Part model, mm, in its own coordinate system. Face numbers are marked on the shaded views. A direction names the side the tool comes from. Coordinates: 2 decimals unless noted, no trailing zeros. Order: outer loops, then holes, each group sorted by start corner. A loop starts at its lowest first (then second) coordinate and runs counter-clockwise, first axis right, second up. Notation, with made-up numbers: (42, 28.5) - (56, 28.5) arc R26 ccw to (56, 50.5) - close; hole circle Ø11 at (70, 3.25). An arc over 180 degrees is marked (long way). Use a Markdown table: item, result. Add a question column.
1) Saw through at D-D on x = 7. List the corners of the cut face in (y, z).
2) Saw through at C-C on y = 3.5. List the corners of the cut face in (x, z), then the cut area to 3 significant figures.
3) Drop flat-ended pins along their axis: P1, Ø2, axis at x = 20, y = 1.5, coming from the +Z side; P2, Ø5, axis at x = 38, y = -2, coming from the -Z side; P3, Ø3, axis at y = -8, z = 0, coming from the +X side; P4, Ø10, axis at x = 22.5, z = -8, coming from the -Y side. Give the stop position or say it passes through.
4) Wall check: L1, parallel to Y at x = 2.55, z = 0; L2, parallel to X at y = -7.5, z = -4; L3, parallel to Z at x = 9.5, y = -1.25. Give the ranges that are in metal, low to high. Write a range as [from, to].
5) Tool access for the marked faces 1, 2 and 3: list every direction of +Z, -Z, +X, -X, +Y, -Y with a clear straight run to the whole face (end or side of a thin tool).
6) Saw through at B-B on y = 0. List the corners of the cut face in (x, z).
7) Saw through at A-A on z = 0. List the corners of the cut face in (x, y), then the cut area to 3 significant figures.
```python
from build123d import *

# Parameters (mm, degrees)
SKETCH1_R           = 1.5
BOSS_EXTRUDE1_DEPTH = 4
SKETCH1_2_R         = 1.5
BOSS_EXTRUDE2_DEPTH = 43
CUT_EXTRUDE1_REACH  = 45
SKETCH2_R           = 1.5


with BuildPart() as part:
    # Sketch1 → Boss-Extrude1 (new body)
    with BuildSketch(Plane(origin=(0, 0, 0), x_dir=(0, 0, -1), z_dir=(1, 0, 0))):
        with BuildLine():
            Line((-4.5, -4.5), (-4.5, 3))
            ThreePointArc((-4.5, 3), (0, 7.5), (4.5, 3))
            Line((4.5, 3), (4.5, -4.5))
            Line((4.5, -4.5), (11.053216354, -9.088611491))
            ThreePointArc((11.053216354, -9.088611491), (0, -14), (-11.053216354, -9.088611491))
            Line((-11.053216354, -9.088611491), (-4.5, -4.5))
        make_face()
        Circle(SKETCH1_R, mode=Mode.SUBTRACT)
    extrude(amount=BOSS_EXTRUDE1_DEPTH)

    # Sketch1<2> → Boss-Extrude2 (add)
    with BuildSketch(Plane(origin=(0, 0, 0), x_dir=(0, 0, -1), z_dir=(1, 0, 0))):
        Circle(SKETCH1_2_R)
    extrude(amount=BOSS_EXTRUDE2_DEPTH)

    # Sketch2 → Cut-Extrude1 (cut, up to next)
    with BuildSketch(Plane.ZY, mode=Mode.PRIVATE) as cut_extrude1_sk1:
        with Locations((0, 3.5)):
            Circle(SKETCH2_R)
    cut_extrude1_tool1 = extrude(cut_extrude1_sk1.sketch, amount=-CUT_EXTRUDE1_REACH, mode=Mode.PRIVATE) & part.part
    add(cut_extrude1_tool1.solids().sort_by_distance((0, 3.5, 0))[0], mode=Mode.SUBTRACT)


solid = part.part
```
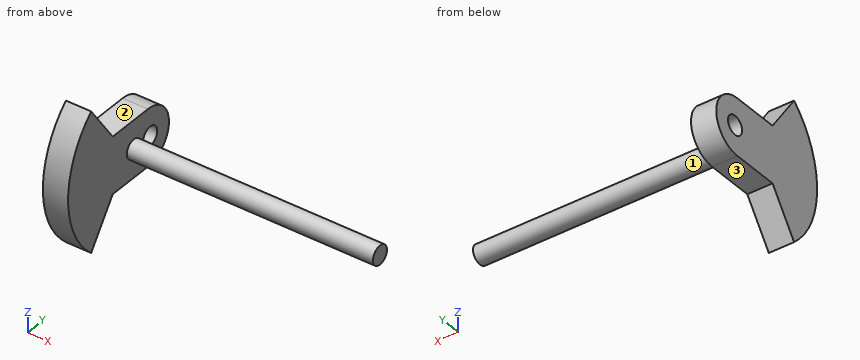
Results are:
| question | item | result |
|---|---|---|
| 1 | outline | circle Ø3 at (0, 0) |
| 2 | outline | (0, -4.47) - (4, -4.47) - (4, -1.5) - (0, -1.5) - close; (0, 1.5) - (4, 1.5) - (4, 4.47) - (0, 4.47) - close |
| 2 | area | 23.8 mm2 |
| 3 | P1 | z = 1.41 |
| 3 | P2 | z = -1.5 |
| 3 | P3 | x = 4 |
| 3 | P4 | through |
| 4 | L1 | [-14, 2], [5, 7.5] |
| 4 | L2 | [0, 4] |
| 4 | L3 | [-0.83, 0.83] |
| 5 | face 1 | +X |
| 5 | face 2 | +Z, +X, -X, +Y |
| 5 | face 3 | -Z, +X, -X, +Y |
| 6 | outline | (0, -4.5) - (4, -4.5) - (4, -1.5) - (43, -1.5) - (43, 1.5) - (4, 1.5) - (4, 4.5) - (0, 4.5) - close |
| 7 | outline | (0, -14) - (4, -14) - (4, -1.5) - (43, -1.5) - (43, 1.5) - (4, 1.5) - (4, 2) - (0, 2) - close; (0, 5) - (4, 5) - (4, 7.5) - (0, 7.5) - close |
| 7 | area | 191 mm2 |
